```python
from build123d import *

# Parameters (mm, degrees)
SKETCH1_W           = 60
SKETCH1_H           = 40
SKETCH1_W_2         = 45
SKETCH1_H_2         = 24.4
BOSS_EXTRUDE1_DEPTH = 5
SKETCH6_W           = 5
SKETCH6_H           = 40
BOSS_EXTRUDE4_DEPTH = 41.5
SKETCH7_W           = 6.5
SKETCH7_H           = 30
BOSS_EXTRUDE5_DEPTH = 25
FILLET2_R           = 2.5
FILLET3_R           = 2.5
CUT_EXTRUDE1_REACH  = 100.093
SKETCH8_R           = 1.025


with BuildPart() as part:
    # Sketch1 → Boss-Extrude1 (new body)
    with BuildSketch(Plane(origin=(0, 0, 0), x_dir=(1, 0, 0), z_dir=(0, 1, 0))):
        with Locations((30, 20)):
            Rectangle(SKETCH1_W, SKETCH1_H)
        with Locations((27.5, 20)):
            Rectangle(SKETCH1_W_2, SKETCH1_H_2, mode=Mode.SUBTRACT)
    extrude(amount=BOSS_EXTRUDE1_DEPTH)

    # Sketch6 → Boss-Extrude4 (add)
    with BuildSketch(Plane.XZ):
        with Locations((2.5, -20)):
            Rectangle(SKETCH6_W, SKETCH6_H)
    extrude(amount=BOSS_EXTRUDE4_DEPTH)

    # Sketch7 → Boss-Extrude5 (add)
    with BuildSketch(Plane(origin=(0, -41.5, 0), x_dir=(-1, 0, 0), z_dir=(0, -1, 0))):
        with Locations((-5.75, 20)):
            Rectangle(SKETCH7_W, SKETCH7_H)
    extrude(amount=BOSS_EXTRUDE5_DEPTH)

    # Fillet2
    fillet2_edges = [part.edges().sort_by_distance(p)[0] for p in [
        (5, -41.5, -20),
        (2.5, -41.5, -20),
    ]]
    fillet(fillet2_edges, radius=FILLET2_R - 0.0001)  # a hair under: the kernel refuses the full size

    # Fillet3
    fillet3_edges = [part.edges().sort_by_distance(p)[0] for p in [
        (2.50005, -41.5, -5),
        (2.50005, -41.5, -35),
        (2.5, -41.5, 0),
        (2.5, -41.5, -40),
    ]]
    fillet(fillet3_edges, radius=FILLET3_R - 0.0001)  # a hair under: the kernel refuses the full size

    # Sketch8 → Cut-Extrude1 (cut, up to next)
    with BuildSketch(Plane(origin=(0, 0, 0), x_dir=(-1, 0, 0), z_dir=(0, -1, 0)), mode=Mode.PRIVATE) as cut_extrude1_sk1:
        with Locations(Location((-52.8, 28.5, 0), (0, 0, 90))):
            Circle(SKETCH8_R)
    cut_extrude1_tool1 = extrude(cut_extrude1_sk1.sketch, amount=-CUT_EXTRUDE1_REACH, mode=Mode.PRIVATE) & part.part
    # Sketch8 → Cut-Extrude1 (cut, up to next)
    with BuildSketch(Plane(origin=(0, 0, 0), x_dir=(-1, 0, 0), z_dir=(0, -1, 0)), mode=Mode.PRIVATE) as cut_extrude1_sk2:
        with Locations(Location((-46.5, 35, 0), (0, 0, 90))):
            Circle(SKETCH8_R)
    cut_extrude1_tool2 = extrude(cut_extrude1_sk2.sketch, amount=-CUT_EXTRUDE1_REACH, mode=Mode.PRIVATE) & part.part
    # Sketch8 → Cut-Extrude1 (cut, up to next)
    with BuildSketch(Plane(origin=(0, 0, 0), x_dir=(-1, 0, 0), z_dir=(0, -1, 0)), mode=Mode.PRIVATE) as cut_extrude1_sk3:
        with Locations(Location((-29.5, 35, 0), (0, 0, 90))):
            Circle(SKETCH8_R)
    cut_extrude1_tool3 = extrude(cut_extrude1_sk3.sketch, amount=-CUT_EXTRUDE1_REACH, mode=Mode.PRIVATE) & part.part
    # Sketch8 → Cut-Extrude1 (cut, up to next)
    with BuildSketch(Plane(origin=(0, 0, 0), x_dir=(-1, 0, 0), z_dir=(0, -1, 0)), mode=Mode.PRIVATE) as cut_extrude1_sk4:
        with Locations(Location((-12.5, 35, 0), (0, 0, 90))):
            Circle(SKETCH8_R)
    cut_extrude1_tool4 = extrude(cut_extrude1_sk4.sketch, amount=-CUT_EXTRUDE1_REACH, mode=Mode.PRIVATE) & part.part
    # Sketch8 → Cut-Extrude1 (cut, up to next)
    with BuildSketch(Plane(origin=(0, 0, 0), x_dir=(-1, 0, 0), z_dir=(0, -1, 0)), mode=Mode.PRIVATE) as cut_extrude1_sk5:
        with Locations(Location((-12.5, 5, 0), (0, 0, 90))):
            Circle(SKETCH8_R)
    cut_extrude1_tool5 = extrude(cut_extrude1_sk5.sketch, amount=-CUT_EXTRUDE1_REACH, mode=Mode.PRIVATE) & part.part
    # Sketch8 → Cut-Extrude1 (cut, up to next)
    with BuildSketch(Plane(origin=(0, 0, 0), x_dir=(-1, 0, 0), z_dir=(0, -1, 0)), mode=Mode.PRIVATE) as cut_extrude1_sk6:
        with Locations(Location((-29.5, 5, 0), (0, 0, 90))):
            Circle(SKETCH8_R)
    cut_extrude1_tool6 = extrude(cut_extrude1_sk6.sketch, amount=-CUT_EXTRUDE1_REACH, mode=Mode.PRIVATE) & part.part
    # Sketch8 → Cut-Extrude1 (cut, up to next)
    with BuildSketch(Plane(origin=(0, 0, 0), x_dir=(-1, 0, 0), z_dir=(0, -1, 0)), mode=Mode.PRIVATE) as cut_extrude1_sk7:
        with Locations(Location((-46.5, 5, 0), (0, 0, 90))):
            Circle(SKETCH8_R)
    cut_extrude1_tool7 = extrude(cut_extrude1_sk7.sketch, amount=-CUT_EXTRUDE1_REACH, mode=Mode.PRIVATE) & part.part
    # Sketch8 → Cut-Extrude1 (cut, up to next)
    with BuildSketch(Plane(origin=(0, 0, 0), x_dir=(-1, 0, 0), z_dir=(0, -1, 0)), mode=Mode.PRIVATE) as cut_extrude1_sk8:
        with Locations(Location((-52.8, 11.5, 0), (0, 0, 90))):
            Circle(SKETCH8_R)
    cut_extrude1_tool8 = extrude(cut_extrude1_sk8.sketch, amount=-CUT_EXTRUDE1_REACH, mode=Mode.PRIVATE) & part.part
    add(cut_extrude1_tool1.solids().sort_by_distance((52.8, 0, -28.5))[0], mode=Mode.SUBTRACT)
    add(cut_extrude1_tool2.solids().sort_by_distance((46.5, 0, -35))[0], mode=Mode.SUBTRACT)
    add(cut_extrude1_tool3.solids().sort_by_distance((29.5, 0, -35))[0], mode=Mode.SUBTRACT)
    add(cut_extrude1_tool4.solids().sort_by_distance((12.5, 0, -35))[0], mode=Mode.SUBTRACT)
    add(cut_extrude1_tool5.solids().sort_by_distance((12.5, 0, -5))[0], mode=Mode.SUBTRACT)
    add(cut_extrude1_tool6.solids().sort_by_distance((29.5, 0, -5))[0], mode=Mode.SUBTRACT)
    add(cut_extrude1_tool7.solids().sort_by_distance((46.5, 0, -5))[0], mode=Mode.SUBTRACT)
    add(cut_extrude1_tool8.solids().sort_by_distance((52.8, 0, -11.5))[0], mode=Mode.SUBTRACT)


solid = part.part
```
For this review, take the finished solid that the model builds, in its own axes (mm). A direction names the side the tool comes from. Coordinates: 2 decimals unless noted, no trailing zeros. Loops run counter-clockwise (first coordinate to the right, second up) from the corner with the lowest first, then second, coordinate; pieces in that order, holes last. Notation, with made-up numbers: (42.5, -26) -> (57.5, -26) arc R15 cw to (57.5, -17) -> close; hole circle Ø9 at (-30.5, 88). An arc over 180 degrees is marked (long way). Return JSON: item names as keys, results as strings. Group by question number.
(1) Consider section D-D, the plane x = 12.5. Give the boundary of the cut face in (y, z) (3 decimals), plus the area to 3 significant figures.
(2) Mouldability with a two-part tool opening along X and no side actions: class faces 1 (the cylindrical face through (12.545, 2.465, -33.976)), 2 (the flat face through (29.6, 5, -33.6)), 3 (the cylindrical face through (30.19, 2.46, -34.24)), 4 (the flat face through (60, 2, -20)) as pulls with the +X half, pulls with the -X half, needs draft (parallel to the pull), parting line crosses it, or undercut.
(3) To check wall thickness, follow L1, parallel to X at y = 3.45, z = -5 (3 decimals); L2, parallel to Z at x = 52, y = 1; L3, parallel to Z at x = 12, y = 2. State the ranges of each line that lie inside material, in increasing order.
(4) Tool access review of faces 5 (the flat face through (9, -54, -20)), 6 (the flat face through (17, 1, 0)), 7 (the flat face through (2.5, -55, -20)): name each direction out of +Z, -Z, +X, -X, +Y, -Y from which nothing blocks a thin tool from reaching the whole face with its end or side.
(5) For pin 1 Ø12 at (y, z) = (-8.5, -32) entering from -X; pin 2 Ø2.5 at (x, z) = (29.5, -5) entering from -Y; pin 3 Ø20 at (y, z) = (-60, -17) entering from +X; pin 4 Ø1.7 at (x, z) = (8, -23) entering from +Y, all flat-tipped, find the tip position at first contact; note any pin that passes through.
(6) Consider section C-C, the plane z = -11.5. Count the separate pieces of the cut face and the enclosed holes in it, plus the area to 3 significant figures.
(7) Consider section B-B, the plane x = 22.5. Give the boundary of the cut face in (y, z), plus the area to 3 significant figures.
Results below:
{
 "1": {"outline": "(0, -40) -> (5, -40) -> (5, -36.025) -> (0, -36.025) -> close; (0, -33.975) -> (5, -33.975) -> (5, -32.2) -> (0, -32.2) -> close; (0, -7.8) -> (5, -7.8) -> (5, -6.025) -> (0, -6.025) -> close; (0, -3.975) -> (5, -3.975) -> (5, 0) -> (0, 0) -> close", "area": "57.5 mm2"},
 "2": {"face 1": "undercut", "face 2": "needs draft", "face 3": "undercut", "face 4": "pulls with the +X half"},
 "3": {"L1": "x = 0 to 11.475, 13.525 to 28.475, 30.525 to 45.475, 47.525 to 60", "L2": "z = -40 to -29.14, -27.86 to -12.14, -10.86 to 0", "L3": "z = -40 to -35.89, -34.11 to -32.2, -7.8 to -5.89, -4.11 to 0"},
 "4": {"face 5": "+Z, -Z, +X, -Y", "face 6": "+Z, +X, -X, +Y, -Y", "face 7": "+Z, -Z, -X, -Y"},
 "5": {"pin 1": "stops at x = 0", "pin 2": "stops at y = 0", "pin 3": "stops at x = 9", "pin 4": "stops at y = -41.48"},
 "6": {"separate pieces": "3", "enclosed holes": "0", "area": "437 mm2"},
 "7": {"outline": "(0, -40) -> (5, -40) -> (5, -32.2) -> (0, -32.2) -> close; (0, -7.8) -> (5, -7.8) -> (5, 0) -> (0, 0) -> close", "area": "78.0 mm2"}
}
